from build123d import *

# Parameters (mm, degrees)
TALADROAVANZADO1_START     = -20
TALADROAVANZADO1_OUTLINE_R = 11.89
TALADROAVANZADO1_DEPTH     = 20


# Read off the part's stored shape, not the designer's step: TaladroAvanzado1
with BuildPart() as part:
    # Croquis1 → Revolución1 (revolve)
    with BuildSketch(Plane(origin=(0, 0, 0), x_dir=(0, 0, -1), z_dir=(1, 0, 0)), mode=Mode.PRIVATE) as revoluci_n1_sk:
        Polygon((0, 0), (0, 28), (10, 28), (10, 21.963), (30, 21.963), (40, 7.5), (40, 0), align=None)
    revolve(revoluci_n1_sk.sketch.rotate(Axis((0, 0, 8.757704884), (0, 0, -1)), 90), axis=Axis((0, 0, 8.757704884), (0, 0, -1)))

    # TaladroAvanzado1 outline → TaladroAvanzado1 (cut)
    with BuildSketch(Plane.XY.offset(TALADROAVANZADO1_START)):
        Circle(TALADROAVANZADO1_OUTLINE_R)
    extrude(amount=TALADROAVANZADO1_DEPTH, mode=Mode.SUBTRACT)


solid = part.part
Check sheet for the modelled part. Datum: model origin and axes. Units: mm. A direction names the side the tool comes from. Coordinates: 2 decimals unless noted, no trailing zeros. Loops run counter-clockwise (first coordinate to the right, second up) from the corner with the lowest first, then second, coordinate; pieces in that order, holes last. Notation, with made-up numbers: (48, 26.25) -> (95, 26.25) arc R23 ccw to (95, 53.25) -> close; hole circle Ø3 at (-11, -17). An arc over 180 degrees is marked (long way). Answer in a Markdown table with one row per item.
1. Release check for a two-part mould opening along Y. For faces 1 (the face through (0, 0, -20)), 2 (the face through (-2.578, -11.607, -10.14)), 3 (the face through (0, 0, -40)), 4 (the face through (7.823, -2.464, -39.514)) record: released by +Y, released by -Y, zero draft, split by the parting line, or undercut.
Check values:
| item | result |
|---|---|
| face 1 | undercut |
| face 2 | undercut |
| face 3 | zero draft |
| face 4 | split by the parting line |
2. Sectioned sample at C-C, the plane z = -6.5. Record the boundary of the cut face in (x, y), then the cut area to 3 significant figures.
Check values:
| item | result |
|---|---|
| outline | circle Ø56 at (0, 0); hole circle Ø23.78 at (0, 0) |
| area | 2,020 mm2 |
3. Go/stop test with flat-tipped pins: pin 1 (8 mm diameter, centred on x = -6, y = -21.5, fed in from +Z); pin 2 (5 mm diameter, centred on x = -4, z = -17, fed in from -Y); pin 3 (12 mm diameter, centred on x = 18.5, z = -36, fed in from -Y); pin 4 (2 mm diameter, centred on x = -18.5, y = 5, fed in from -Z). Record where each tip stops, or that it passes through.
Check values:
| item | result |
|---|---|
| pin 1 | stops at z = 0 |
| pin 2 | stops at y = -21.91 |
| pin 3 | stops at y = -13.89 |
| pin 4 | stops at z = -32.63 |
4. Material ranges on line 1 along Y through (x, z) = (0, -6); line 2 along Z through (x, y) = (21, 14); line 3 along X through (y, z) = (0.5, -21.5), recorded low to high. Write a range as [from, to].
Check values:
| item | result |
|---|---|
| line 1 | y = [-28, -11.89], [11.89, 28] |
| line 2 | z = [-10, 0] |
| line 3 | x = [-21.96, 21.96] |
5. Access from +Z, -Z, +X, -X, +Y, -Y to the whole of each face (thin tool, end or side, straight path). Record for faces 5 (the face through (-17.4, 13.4, -20.1)), 6 (the face through (12.92, 24.84, -5.07)).
Check values:
| item | result |
|---|---|
| face 5 | -Z |
| face 6 | +Z, -Z |
6. Sectioned sample at D-D, the plane z = -33. Record the boundary of the cut face in (x, y).
Check values:
| item | result |
|---|---|
| outline | circle Ø35.25 at (0, 0) |
7. Sectioned sample at A-A, the plane x = 0. Record the boundary of the cut face in (y, z), then the cut area to 3 significant figures.
Check values:
| item | result |
|---|---|
| outline | (-28, -10) -> (-21.96, -10) -> (-21.96, -30) -> (-7.5, -40) -> (7.5, -40) -> (21.96, -30) -> (21.96, -10) -> (28, -10) -> (28, 0) -> (11.89, 0) -> (11.89, -20) -> (-11.89, -20) -> (-11.89, 0) -> (-28, 0) -> close |
| area | 1,260 mm2 |
